Can you work these out from the drawing? Everything is in mm from the part's minimum corner. A direction names the side the tool comes from. Give positions to 0.01 mm unless a question says otherwise; leave off trailing zeros. Write each loop counter-clockwise with the first axis right and the second up, starting at its lowest first coordinate (ties: lowest second). Pieces come first, ordered by that corner, then holes. Notation, with made-up numbers: (32, 55.5) -> (72, 55.5) arc R15 ccw to (72, 66.5) -> close; hole circle Ø11 at (-33, 13). An arc over 180 degrees is marked (long way). Use one line per item in the form item = value.
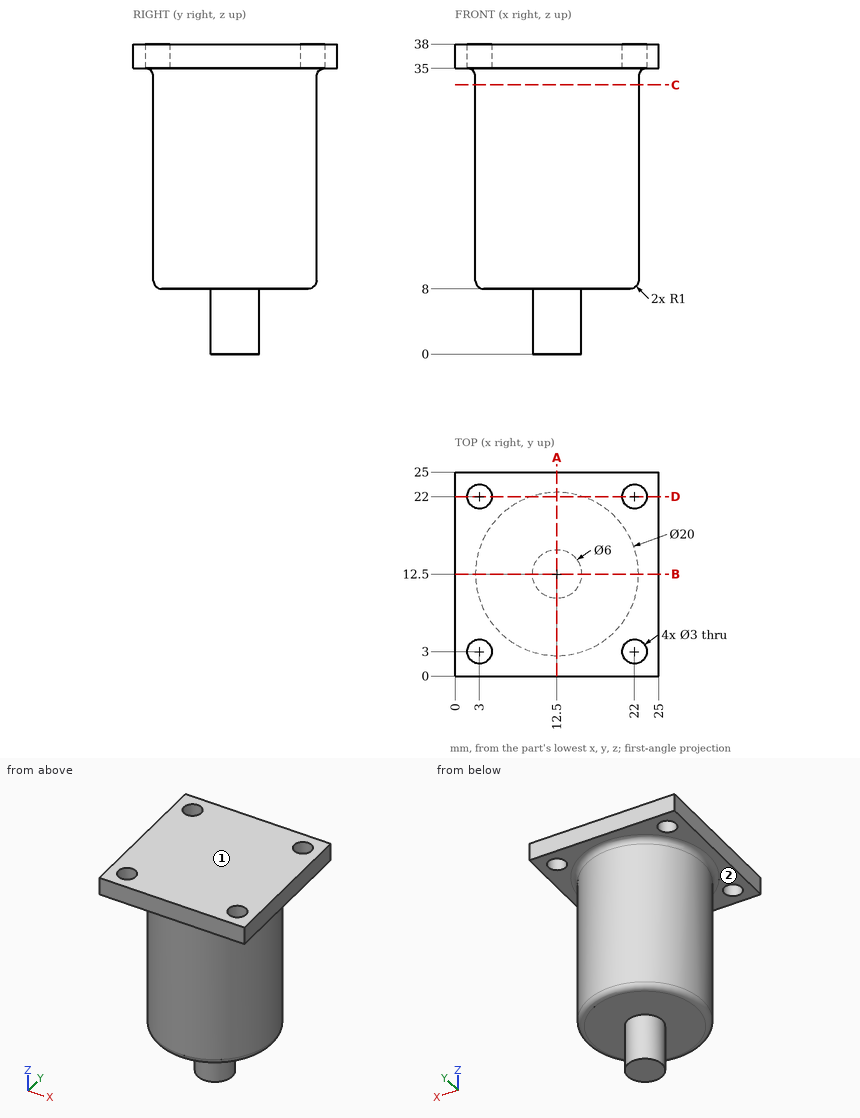
Q1. I want a section at D-D, the plane y = 22. Count the separate pieces of the cut face and the enclosed holes in it, and give its area (3 significant figures).
Result set:
separate_pieces = 3
enclosed_holes = 0
area = 225 mm2
Q2. Will these pins go through, and if not, where does the flat tip stop? pin 1 Ø2.5 at (x, y) = (3, 22) entering from -Z; pin 2 Ø5 at (x, z) = (20.5, 10.5) entering from -Y; pin 3 Ø2 at (y, z) = (13.5, 15) entering from -X; pin 4 Ø1.5 at (x, y) = (10.5, 21.5) entering from -Z.
Result set:
pin_1 = through
pin_2 = 4.15
pin_3 = 2.5
pin_4 = 8
Q3. I want a section at C-C, the plane z = 33. Write out the boundary of the cut face in (x, y), and give its area (3 significant figures).
Result set:
outline = circle Ø20 at (12.5, 12.5)
area = 314 mm2
Q4. Which directions (+Z, -Z, +X, -X, +Y, -Y) give clear straight access to the entire face, cutting with the end or side of a thin tool? Please do the marked faces 1 and 2.
Result set:
face_1 = +Z, +X, -X, +Y, -Y
face_2 = -Z
Q5. If I drill on line 1 along Y through (x, z) = (3, 36.2); line 2 along Z through (x, y) = (8, 13.5); line 3 along Z through (x, y) = (20.5, 3.5), over which ranges is the centre line in solid material (lowest first)? Write a range as from..to.
Result set:
line_1 = 0..1.5, 4.5..20.5, 23.5..25
line_2 = 8..38
line_3 = 35..38
Q6. I want a section at A-A, the plane x = 12.5. Write out the boundary of the cut face in (y, z).
Result set:
outline = (0, 35) -> (1.5, 35) arc R1 cw to (2.5, 34) -> (2.5, 9) arc R1 ccw to (3.5, 8) -> (9.5, 8) -> (9.5, 0) -> (15.5, 0) -> (15.5, 8) -> (21.5, 8) arc R1 ccw to (22.5, 9) -> (22.5, 34) arc R1 cw to (23.5, 35) -> (25, 35) -> (25, 38) -> (0, 38) -> close
